```python
from build123d import *

# Parameters (mm, degrees)
SKETCH1_R           = 6
BOSS_EXTRUDE2_DEPTH = 5
CHAMFER1_SIZE       = 1


with BuildPart() as part:
    # Sketch1 → Boss-Extrude2 (new body, symmetric)
    with BuildSketch(Plane(origin=(0, 0, 0), x_dir=(0, 0, -1), z_dir=(1, 0, 0))):
        Circle(SKETCH1_R)
    extrude(amount=BOSS_EXTRUDE2_DEPTH, both=True)

    # Sketch5 → M6x1.0 Tapped Hole1 (revolve, cut)
    with BuildSketch(Plane(origin=(-5, 0, 0), x_dir=(0, 0, 1), z_dir=(0, 1, 0))):
        Polygon((0, 0), (0, 7.502151548), (2.5, 6), (2.5, 0), align=None)
    revolve(axis=Axis((-11.35, 0, 0), (1, 0, 0)), mode=Mode.SUBTRACT)

    # Chamfer1
    chamfer1_edges = [part.edges().sort_by_distance(p)[0] for p in [
        (5, 0, 6),
    ]]
    chamfer(chamfer1_edges, length=CHAMFER1_SIZE)


solid = part.part
```
Part model, mm, in its own coordinate system. A direction names the side the tool comes from. Coordinates: 2 decimals unless noted, no trailing zeros. Loops run counter-clockwise (first coordinate to the right, second up) from the corner with the lowest first, then second, coordinate; pieces in that order, holes last. Notation, with made-up numbers: (-13.5, 70) - (11.5, 70) arc R15 ccw to (11.5, 78) - close; hole circle Ø5 at (-17, 61). An arc over 180 degrees is marked (long way). Write item = value, one per line. Start each with the question number.
Item 1: 3-axis set-ups, long thin cutter, end or side, ignore diameter. For faces 4 (the flat face through (-5, 0, -3)), 5 (the cylindrical face through (-2.04, 2.44, -0.54)): which of +Z, -Z, +X, -X, +Y, -Y reach the whole face in a straight line?
Item 2: Wall check: L1, parallel to Y at x = -3.3, z = 0; L2, parallel to Z at x = -2, y = -1; L3, parallel to Z at x = 2.75, y = -1. Give the ranges that are in metal, low to high. Write a range as from..to.
Item 3: Mould opens along Z. For faces 1 (the conical face through (2.241, 0.424, -0.094)), 2 (the cylindrical face through (0, 0, 6)), 3 (the flat face through (5, 0, 0)) say: released by +Z, released by -Z, zero draft, split by the parting line, or undercut.
Item 4: Cut at B-B, the plane x = 1.25. Give the cut face in (y, z), and give its area (3 significant figures).
Item 5: Cut at A-A, the plane x = 0.25. Give the cut face in (y, z), and give its area (3 significant figures).
Item 6: Flat gauge pins, fed straight in: pin 1 Ø1.5 at (x, y) = (-2, -2) entering from +Z; pin 2 Ø1 at (x, y) = (4, 4.5) entering from -Z; pin 3 Ø1.5 at (x, y) = (-3, 1) entering from +Z. Where does each tip first touch, or does it go through?
The answers:
q1.face_4 = +Z, -Z, -X, +Y, -Y
q1.face_5 = -X
q2.L1 = -6..-2.5, 2.5..6
q2.L2 = -5.92..-2.29, 2.29..5.92
q2.L3 = -5.92..5.92
q3.face_1 = undercut
q3.face_2 = split by the parting line
q3.face_3 = zero draft
q4.outline = circle Ø12 at (0, 0); hole circle Ø4.17 at (0, 0)
q4.area = 99.5 mm2
q5.outline = circle Ø12 at (0, 0); hole circle Ø5 at (0, 0)
q5.area = 93.5 mm2
q6.pin_1 = 5.87
q6.pin_2 = -4.47
q6.pin_3 = 5.99
